```python
from build123d import *

# Parameters (mm, degrees)
F4_R = 5.99999


# Not quite as in the source:
# - a fillet or chamfer is up to 0.001 mm smaller than in the source, because OpenCascade refuses the exact size


with BuildPart() as f1:
    # F0 (on Front) → F1 (revolve)
    with BuildSketch(Plane.XZ):
        with BuildLine():
            Line((0, 31), (0, 0))
            Line((0, 0), (88, 0))
            Line((88, 0), (88, 15))
            Line((88, 15), (85, 15))
            Line((85, 15), (85, 20))
            Line((85, 20), (68, 20))
            Line((68, 20), (68, 31))
            Line((68, 31), (56, 31))
            ThreePointArc((56, 31), (50, 25), (44, 31))
            Line((44, 31), (0, 31))
        make_face()
    revolve(axis=Axis((45.4589584282, 0, 0), (1, 0, 0)))

    # F2 (on Front) → F3 (revolve, cut)
    with BuildSketch(Plane.XZ):
        Polygon((0, 25), (0, 0), (88, 0), (88, 6), (30, 6), (30, 16), (22, 16), (22, 20.5), (19, 20.5), (19, 12.5), (12, 12.5), (12, 16), (1.5, 16), (1.5, 25), align=None)
    revolve(axis=Axis((-7.9182099137, 0, 0), (-1, 0, 0)), mode=Mode.SUBTRACT)

    # F4 (radius 6 in the source; OpenCascade refuses exactly that, so slightly less here)
    f4_edges = [f1.edges().sort_by_distance(p)[0] for p in [
        (0, 0, -31),
    ]]
    fillet(f4_edges, radius=F4_R)


solid = f1.part
```
Geometry: final body of the model. Coordinates: model frame, mm. A direction names the side the tool comes from. Round coordinates to 2 decimals unless told otherwise and drop trailing zeros. Order: outer loops, then holes, each group sorted by start corner. A loop starts at its lowest first (then second) coordinate and runs counter-clockwise, first axis right, second up. Notation, with made-up numbers: (63.25, 5) - (88.25, 5) arc R17 cw to (88.25, 15) - close; hole circle Ø6 at (-36.75, 11.25). An arc over 180 degrees is marked (long way). Use CSV: the item, a comma, the result in double quotes. Start each with the question number.
Q1. First-contact query: pin 1 (18.5 mm diameter, centred on y = 4, z = 2.5, fed in from +X); pin 2 (5 mm diameter, centred on x = 44.5, y = 24.5, fed in from +Z); pin 3 (10 mm diameter, centred on y = -18.5, z = 19, fed in from +X); pin 4 (10 mm diameter, centred on x = 74, z = -21, fed in from -Y). Flat tips, straight axial feed; report the tip coordinate or a pass-through.
Q2. Access query for faces 1 (the face through (68, 20.2, 0.4)), 2 (the face through (15.451, 3.755, 11.923)), 3 (the face through (59, 0, -6)), 4 (the face through (19, -9, -9)). Directions: +Z, -Z, +X, -X, +Y, -Y. A direction counts if a zero-diameter tool reaches every point of the face in a straight line with its end or side. Return the directions, or none.
Q3. Section query A-A (x = 10). Return loops of the section in (y, z), and give its area (3 significant figures).
Q4. Section query B-B (x = 82.5). Return loops of the section in (y, z), and give its area (3 significant figures).
Q5. Material intervals for line 1 along X through (y, z) = (-7, -11.5); line 2 along Y through (x, z) = (15, 0); line 3 along X through (y, z) = (4, -16), sorted ascending. Write a range as from..to.
Q6. Mould query, pull axis Y, two halves, no side actions, for faces 5 (the face through (88, 6.5, 0.2)), 6 (the face through (6.68, -15.62, -3.47)), 7 (the face through (61.916, -30.736, -4.036)). Classes: +Y half, -Y half, draft (parallel to the pull), parting line (faces both ways), or undercut.
Result set:
1,pin 1,"stops at x = 88"
1,pin 2,"stops at z = 21.79"
1,pin 3,"stops at x = 68"
1,pin 4,"stops at y = -12"
2,face 1,"+X"
2,face 2,"-X"
2,face 3,"+X, -X"
2,face 4,"none"
3,outline,"circle Ø62 at (0, 0); hole circle Ø32 at (0, 0)"
3,area,"2,210 mm2"
4,outline,"circle Ø40 at (0, 0); hole circle Ø12 at (0, 0)"
4,area,"1,140 mm2"
5,line 1,"x = 12..19, 30..88"
5,line 2,"y = -31..-12.5, 12.5..31"
5,line 3,"x = 1.5..19, 22..85"
6,face 5,"draft"
6,face 6,"undercut"
6,face 7,"parting line"
